Can you work these out from the model? Positions are in its coordinate system, mm. Coordinates: 2 decimals unless noted, no trailing zeros. Write each loop counter-clockwise with the first axis right and the second up, starting at its lowest first coordinate (ties: lowest second). Pieces come first, ordered by that corner, then holes.
```python
from build123d import *

# Parameters (mm, degrees)
F0_R     = 10.5
F1_DEPTH = 11
F2_R     = 3.5
F3_DEPTH = 3
F4_SIZE  = 5


with BuildPart() as f1:
    # F0 (on Top) → F1 (new body)
    with BuildSketch(Plane.XY):
        Circle(F0_R)
    extrude(amount=F1_DEPTH)

    # F2 (on face) → F3 (cut)
    with BuildSketch(Plane.XY.offset(11)):
        Circle(F2_R)
    extrude(amount=-F3_DEPTH, mode=Mode.SUBTRACT)

    # F4
    f4_edges = [f1.edges().sort_by_distance(p)[0] for p in [
        (-10.5, 0, 0),
    ]]
    chamfer(f4_edges, length=F4_SIZE)


solid = f1.part
```
1. We'd pull the mould along Y, two halves only. Please class faces 1 (the face through (-1.245, -5.606, 0.243)), 2 (the face through (0, 0, 8)), 3 (the face through (5, 0, 11)), 4 (the face through (3.233, -1.341, 9.521)): released by +Y, released by -Y, zero draft, split by the parting line, or undercut.
2. If we section it at D-D, the plane z = 4: List the corners of the cut face in (x, y) for me, plus the area to 3 significant figures.
3. If we section it at C-C, the plane z = 6: List the corners of the cut face in (x, y) for me, plus the area to 3 significant figures.
4. I'm going to push flat-ended pins straight in: P1, Ø2, axis at x = 1.5, y = -0.5, coming from the +Z side; P2, Ø3, axis at x = -3.5, z = 1.5, coming from the +Y side; P3, Ø1, axis at x = 6, z = 4.5, coming from the +Y side. Where does each tip first touch, or does it pass through?
5. If we section it at A-A, the plane x = 0: List the corners of the cut face in (y, z) for me.
6. If I drill on L1, parallel to Y at x = 0, z = 8.65; L2, parallel to Y at x = 5.5, z = 1.25; L3, parallel to Y at x = 5.25, z = 4.25, over which ranges is the centre line in solid material (lowest first)?
Answers:
1. face 1: split by the parting line
1. face 2: undercut
1. face 3: zero draft
1. face 4: undercut
2. outline: circle Ø19 at (0, 0)
2. area: 284 mm2
3. outline: circle Ø21 at (0, 0)
3. area: 346 mm2
4. P1: stops at z = 8
4. P2: stops at y = 7.86
4. P3: stops at y = 8.71
5. outline: (-10.5, 5) - (-5.5, 0) - (5.5, 0) - (10.5, 5) - (10.5, 11) - (3.5, 11) - (3.5, 8) - (-3.5, 8) - (-3.5, 11) - (-10.5, 11) - close
6. L1: y = -10.5 to -3.5, 3.5 to 10.5
6. L2: y = -3.91 to 3.91
6. L3: y = -8.22 to 8.22
